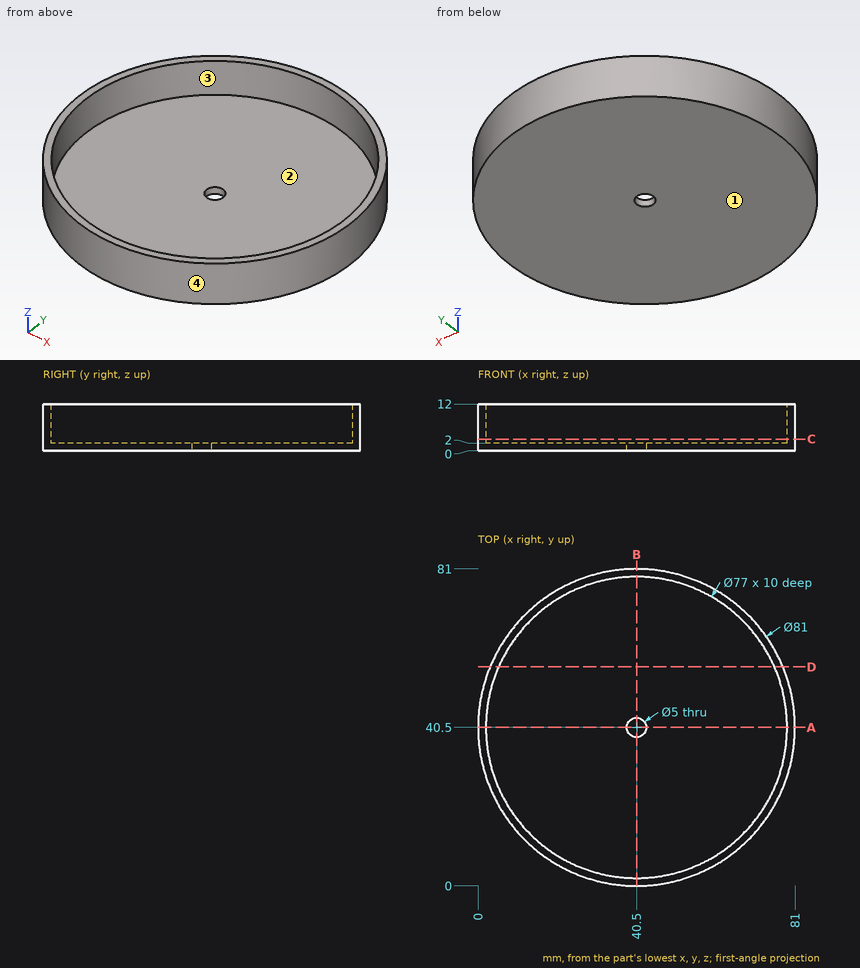
Input: dimensioned drawing with shaded views. Units: mm. Origin: part minimum x, y, z. Coordinates: 2 decimals unless noted, no trailing zeros. Order: outer loops, then holes, each group sorted by start corner. A loop starts at its lowest first (then second) coordinate and runs counter-clockwise, first axis right, second up.
Item 1: Section query A-A (y = 40.5). Output: boundary loops of the cut face in (x, z), then the cut area to 3 significant figures.
Answer:
outline: (0, 0) - (38, 0) - (38, 2) - (2, 2) - (2, 12) - (0, 12) - close; (43, 0) - (81, 0) - (81, 12) - (79, 12) - (79, 2) - (43, 2) - close
area: 192 mm2
Item 2: Draft query along Y for the marked faces 1, 2, 3 and 4. Return one class per face: released by +Y, released by -Y, zero draft, split by the parting line, or undercut.
Answer:
face 1: zero draft
face 2: undercut
face 3: undercut
face 4: split by the parting line
Item 3: Section query D-D (y = 56). Output: boundary loops of the cut face in (x, z), then the cut area to 3 significant figures.
Answer:
outline: (3.08, 0) - (77.92, 0) - (77.92, 12) - (75.74, 12) - (75.74, 2) - (5.26, 2) - (5.26, 12) - (3.08, 12) - close
area: 193 mm2
Item 4: Material intervals for line 1 along Y through (x, z) = (40.5, 9.25); line 2 along Z through (x, y) = (55, 22.5); line 3 along X through (y, z) = (56.5, 6.75), sorted ascending.
Answer:
line 1: y = 0 to 2, 79 to 81
line 2: z = 0 to 2
line 3: x = 3.29 to 5.48, 75.52 to 77.71
Item 5: Contact query for flat-ended pins moving along their axis: P1, Ø5, axis at y = 12.5, z = 11, coming from the -X side; P2, Ø4, axis at x = 27.5, y = 45, coming from the +Z side; P3, Ø12, axis at x = 71, y = 69.5, coming from the -Z side; P4, Ø2, axis at y = 47, z = 3, coming from the -X side. Output: stop coordinate, or through.
Answer:
P1: stops at x = 9.04
P2: stops at z = 2
P3: stops at z = 0
P4: stops at x = 0.38
Item 6: Section query C-C (z = 3). Output: boundary loops of the cut face in (x, y).
Answer:
outline: circle Ø81 at (40.5, 40.5); hole circle Ø77 at (40.5, 40.5)
